from build123d import *

# Parameters (mm, degrees)
F1_DEPTH = 2133.6


with BuildPart() as f1:
    # F0 (on Front) → F1 (new body)
    with BuildSketch(Plane.XZ):
        with BuildLine():
            Line((24.488532, 35.02659), (-27.581468, 35.02659))
            ThreePointArc((-27.581468, 35.02659), (-29.377519, 34.282641), (-30.121468, 32.48659))
            Line((-30.121468, 32.48659), (-30.121468, -19.58341))
            ThreePointArc((-30.121468, -19.58341), (-29.377519, -21.379462), (-27.581468, -22.12341))
            Line((-27.581468, -22.12341), (24.488532, -22.12341))
            ThreePointArc((24.488532, -22.12341), (26.284584, -21.379462), (27.028532, -19.58341))
            Line((27.028532, -19.58341), (27.028532, 32.48659))
            ThreePointArc((27.028532, 32.48659), (26.284584, 34.282641), (24.488532, 35.02659))
        make_face()
        with BuildLine():
            ThreePointArc((-23.771468, 26.13659), (-23.027519, 27.932641), (-21.231468, 28.67659))
            Line((-21.231468, 28.67659), (20.678532, 28.67659))
            Line((20.678532, 28.67659), (20.678532, -13.23341))
            ThreePointArc((20.678532, -13.23341), (19.934584, -15.029462), (18.138532, -15.77341))
            Line((18.138532, -15.77341), (-21.231468, -15.77341))
            ThreePointArc((-21.231468, -15.77341), (-23.027519, -15.029462), (-23.771468, -13.23341))
            Line((-23.771468, -13.23341), (-23.771468, 26.13659))
        make_face(mode=Mode.SUBTRACT)
    extrude(amount=F1_DEPTH)


solid = f1.part
Geometry: final body of the model. Coordinates: model frame, mm. A direction names the side the tool comes from. Give positions to 0.01 mm unless a question says otherwise; leave off trailing zeros. Order: outer loops, then holes, each group sorted by start corner. A loop starts at its lowest first (then second) coordinate and runs counter-clockwise, first axis right, second up. Notation, with made-up numbers: (47, 61.5) -> (78, 61.5) arc R12 ccw to (78, 82.5) -> close; hole circle Ø8 at (14, 7.5). An arc over 180 degrees is marked (long way). Answer as a JSON object with one key per item and string values.
Q1. Access query for faces 1 (the flat face through (-1, -1052, 28.677)), 2 (the flat face through (-2, -1052, -22.123)). Directions: +Z, -Z, +X, -X, +Y, -Y. A direction counts if a zero-diameter tool reaches every point of the face in a straight line with its end or side. Return the directions, or none.
Entries:
{"face 1": "+Y, -Y", "face 2": "-Z, +X, -X, +Y, -Y"}
Q2. First-contact query: pin 1 (10 mm diameter, centred on x = 16, z = 19, fed in from -Y). Flat tip, straight axial feed; report the tip coordinate or a pass-through.
Entries:
{"pin 1": "stops at y = -2133.6"}
Q3. Section B-B (x = 8). Output: boundary loops of the cut face in (y, z), plus the area to 3 significant figures.
Entries:
{"outline": "(-2133.6, -22.12) -> (0, -22.12) -> (0, -15.77) -> (-2133.6, -15.77) -> close; (-2133.6, 28.68) -> (0, 28.68) -> (0, 35.03) -> (-2133.6, 35.03) -> close", "area": "27,100 mm^2"}
Q4. Material intervals for probe 1 along Z at (x, y) = (-2, -1672); probe 2 along X at (y, z) = (-1416, -12.5); probe 3 along X at (y, z) = (-1187, 27), sorted ascending.
Entries:
{"probe 1": "z = -22.12 to -15.77, 28.68 to 35.03", "probe 2": "x = -30.12 to -23.77, 20.68 to 27.03", "probe 3": "x = -30.12 to -23.62, 20.68 to 27.03"}
Q5. Section C-C (y = -1154). Output: boundary loops of the cut face in (x, z), plus the area to 3 significant figures.
Entries:
{"outline": "(-30.12, -19.58) arc R2.54 ccw to (-27.58, -22.12) -> (24.49, -22.12) arc R2.54 ccw to (27.03, -19.58) -> (27.03, 32.49) arc R2.54 ccw to (24.49, 35.03) -> (-27.58, 35.03) arc R2.54 ccw to (-30.12, 32.49) -> close; hole (-23.77, -13.23) arc R2.54 ccw to (-21.23, -15.77) -> (18.14, -15.77) arc R2.54 ccw to (20.68, -13.23) -> (20.68, 28.68) -> (-21.23, 28.68) arc R2.54 ccw to (-23.77, 26.14) -> close", "area": "1,290 mm^2"}
Q6. Section A-A (z = 9). Output: boundary loops of the cut face in (x, y).
Entries:
{"outline": "(-30.12, -2133.6) -> (-23.77, -2133.6) -> (-23.77, 0) -> (-30.12, 0) -> close; (20.68, -2133.6) -> (27.03, -2133.6) -> (27.03, 0) -> (20.68, 0) -> close"}
Q7. Draft query along Z for faces 3 (the flat face through (-1, -1052, 35.027)), 4 (the flat face through (-23.771, -1052, 6)), 5 (the flat face through (27.029, -1052, 6)). Return one class per face: released by +Z, released by -Z, zero draft, split by the parting line, or undercut.
Entries:
{"face 3": "released by +Z", "face 4": "undercut", "face 5": "zero draft"}
